```python
from build123d import *

# Parameters (mm, degrees)
SKETCH1_W           = 30
SKETCH1_H           = 13
BOSS_EXTRUDE2_DEPTH = 3
BOSS_EXTRUDE3_DEPTH = 65
SKETCH5_R           = 1.5
CUT_EXTRUDE3_DEPTH  = 13
SKETCH6_R           = 1.5
BOSS_EXTRUDE4_DEPTH = 3
SKETCH7_W           = 5.6
SKETCH7_H           = 3.1
CUT_EXTRUDE4_DEPTH  = 6


with BuildPart() as part:
    # Sketch1 → Boss-Extrude2 (new body)
    with BuildSketch(Plane.XY):
        with BuildLine():
            Line((0, 0), (50, 0))
            Line((50, 0), (50, 4.071593084))
            ThreePointArc((50, 4.071593084), (44.142135624, 18.213728707), (30, 24.071593084))
            Line((30, 24.071593084), (20, 24.071593084))
            ThreePointArc((20, 24.071593084), (5.857864376, 18.213728707), (0, 4.071593084))
            Line((0, 4.071593084), (0, 0))
        make_face()
        with Locations((25, 10.1)):
            Rectangle(SKETCH1_W, SKETCH1_H, mode=Mode.SUBTRACT)
    extrude(amount=BOSS_EXTRUDE2_DEPTH)

    # Sketch1_4 → Boss-Extrude3 (add)
    with BuildSketch(Plane.XY):
        with BuildLine():
            Line((0, 4.071593084), (0, 0))
            Line((0, 0), (50, 0))
            Line((50, 0), (50, 4.071593084))
            ThreePointArc((50, 4.071593084), (44.142135624, 18.213728707), (30, 24.071593084))
            Line((30, 24.071593084), (20, 24.071593084))
            ThreePointArc((20, 24.071593084), (5.857864376, 18.213728707), (0, 4.071593084))
        make_face()
        with BuildLine():
            Line((10, 11.543086969), (10, 16.6))
            Line((10, 16.6), (40, 16.6))
            Line((40, 16.6), (40, 11.543086969))
            ThreePointArc((40, 11.543086969), (45.95, 10.1), (40, 8.656913031))
            Line((40, 8.656913031), (40, 3.6))
            Line((40, 3.6), (25, 3.6))
            Line((25, 3.6), (10, 3.6))
            Line((10, 3.6), (10, 8.656913031))
            ThreePointArc((10, 8.656913031), (4.05, 10.1), (10, 11.543086969))
        make_face(mode=Mode.SUBTRACT)
    extrude(amount=BOSS_EXTRUDE3_DEPTH)

    # Sketch5 → Cut-Extrude3 (cut)
    with BuildSketch(Plane.XY.offset(65)):
        with Locations((5.5, 3)):
            Circle(SKETCH5_R)
        with Locations((44.5, 3)):
            Circle(SKETCH5_R)
    extrude(amount=-CUT_EXTRUDE3_DEPTH, mode=Mode.SUBTRACT)

    # Sketch6 → Boss-Extrude4 (add)
    # profile 1 of 2: a face of its own
    with BuildSketch(Plane(origin=(0, 0, 0), x_dir=(-1, 0, 0), z_dir=(0, -1, 0))):
        with BuildLine():
            Line((-60, -21.270803163), (-60, -57.567716257))
            ThreePointArc((-60, -57.567716257), (-55.406345217, -60.42004806), (-50, -60.514347456))
            Line((-50, -60.514347456), (-50, 0))
            ThreePointArc((-50, 0), (-52.87596668, -11.633969103), (-60, -21.270803163))
        make_face()
        with Locations(Location((-55, -53.75, 0), (0, 0, 90))):
            Circle(SKETCH6_R, mode=Mode.SUBTRACT)
        with Locations(Location((-55, -21.270803163, 0), (0, 0, 270))):
            Circle(SKETCH6_R, mode=Mode.SUBTRACT)
    # profile 2 of 2: a face of its own
    with BuildSketch(Plane(origin=(0, 0, 0), x_dir=(-1, 0, 0), z_dir=(0, -1, 0))):
        with BuildLine():
            Line((0, -60.514347456), (0, 0))
            ThreePointArc((0, 0), (2.87596668, -11.633969103), (10, -21.270803163))
            Line((10, -21.270803163), (10, -57.567716257))
            ThreePointArc((10, -57.567716257), (5.406345217, -60.42004806), (0, -60.514347456))
        make_face()
        with Locations(Location((5, -21.270803163, 0), (0, 0, 90))):
            Circle(SKETCH6_R, mode=Mode.SUBTRACT)
        with Locations(Location((5, -53.75, 0), (0, 0, 270))):
            Circle(SKETCH6_R, mode=Mode.SUBTRACT)
    extrude(amount=-BOSS_EXTRUDE4_DEPTH)

    # Sketch7 → Cut-Extrude4 (cut)
    with BuildSketch(Plane.XZ):
        with Locations((44.5, 60)):
            Rectangle(SKETCH7_W, SKETCH7_H)
        with Locations((5.5, 60)):
            Rectangle(SKETCH7_W, SKETCH7_H)
    extrude(amount=-CUT_EXTRUDE4_DEPTH, mode=Mode.SUBTRACT)


solid = part.part
```
Here's how the part is built. I have some questions about the finished solid (model axes, mm). A direction names the side the tool comes from. Coordinates: 2 decimals unless noted, no trailing zeros. Order: outer loops, then holes, each group sorted by start corner. A loop starts at its lowest first (then second) coordinate and runs counter-clockwise, first axis right, second up.
1) Will these pins go through, and if not, where does the flat tip stop? pin 1 (1.5 mm diameter, centred on y = 20, z = 51.5, fed in from -X); pin 2 (0.9 mm diameter, centred on y = 4, z = 59.5, fed in from +X); pin 3 (10 mm diameter, centred on y = 13.5, z = 18.5, fed in from +X); pin 4 (2.5 mm diameter, centred on x = 5.5, y = 3, fed in from -Z).
2) Which directions (+Z, -Z, +X, -X, +Y, -Y) give clear straight access to the entire face, cutting with the end or side of a thin tool? Please do faces 1 (the face through (2.7, 3, 60)), 2 (the face through (7, 10, 3)), 3 (the face through (10, 7, 32)).
3) I need wall thicknesses on line 1 (Y direction, x = 27, z = 35); line 2 (X direction, y = 13, z = 21); line 3 (X direction, y = 4.25, z = 10.5). Which ranges of each line are inside material? Lowest first, please.
4) Imagine slicing it at C-C on z = 10. List the corners of the cut face in (x, y) for me.
5) Imagine slicing it at D-D on x = -5. List the corners of the cut face in (y, z) for me, and give its area (3 significant figures).
6) Imagine slicing it at B-B on y = 10.1. List the corners of the cut face in (x, z) for me, and give its area (3 significant figures).
7) We'd pull the mould along X, two halves only. Please class faces 4 (the face through (-5, 3, 37)), 5 (the face through (55.48, 1.48, 60.4)), 6 (the face through (44.297, 18.057, 32.045)): +X half, -X half, draft (parallel to the pull), parting line (faces both ways), or undercut.
8) Imagine slicing it at A-A on x = 17.5. List the corners of the cut face in (y, z) for me, and give its area (3 significant figures).
Response values:
1. pin 1: stops at x = 6.98
1. pin 2: stops at x = 50
1. pin 3: stops at x = 49.5
1. pin 4: stops at z = 0
2. face 1: -Y
2. face 2: +Z
2. face 3: +Z, -Z
3. line 1: y = 0 to 3.6, 16.6 to 24.07
3. line 2: x = 2.1 to 5.97, 8.43 to 10, 40 to 41.57, 44.03 to 47.9
3. line 3: x = 0 to 10, 40 to 50
4. outline: (-2.17, 0) - (52.17, 0) - (52.17, 3) - (50, 3) - (50, 4.07) arc R20 ccw to (30, 24.07) - (20, 24.07) arc R20 ccw to (0, 4.07) - (0, 3) - (-2.17, 3) - close; hole (10, 3.6) - (40, 3.6) - (40, 8.66) arc R3.15 ccw (long way) to (40, 11.54) - (40, 16.6) - (10, 16.6) - (10, 11.54) arc R3.15 ccw (long way) to (10, 8.66) - close
5. outline: (0, 15.43) - (3, 15.43) - (3, 19.77) - (0, 19.77) - close; (0, 22.77) - (3, 22.77) - (3, 52.25) - (0, 52.25) - close; (0, 55.25) - (3, 55.25) - (3, 60.53) - (0, 60.53) - close
5. area: 117 mm2
6. outline: (0.93, 0) - (10, 0) - (10, 3) - (4.05, 3) - (4.05, 65) - (0.93, 65) - close; (40, 0) - (49.07, 0) - (49.07, 65) - (45.95, 65) - (45.95, 3) - (40, 3) - close
6. area: 441 mm2
7. face 4: draft
7. face 5: undercut
7. face 6: +X half
8. outline: (0, 0) - (3.6, 0) - (3.6, 65) - (0, 65) - close; (16.6, 0) - (23.91, 0) - (23.91, 65) - (16.6, 65) - close
8. area: 709 mm2
